Geometry check sheet. Reference: the model listing, model coordinates, mm. A direction names the side the tool comes from. Coordinates: 2 decimals unless noted, no trailing zeros. Order: outer loops, then holes, each group sorted by start corner. A loop starts at its lowest first (then second) coordinate and runs counter-clockwise, first axis right, second up. Notation, with made-up numbers: (5, -1.75) - (55, -1.75) arc R7 ccw to (55, 3.25) - close; hole circle Ø7 at (6.5, -23). An arc over 180 degrees is marked (long way). Return JSON: item names as keys, results as strings. Group by question number.
Item 1: Section check A-A on y = 12.5. Enter the section's corners in (x, z), then the cut area to 3 significant figures.
Item 2: Section check B-B on x = -63.5. Enter the section's corners in (y, z), then the cut area to 3 significant figures.
Item 3: Section check D-D on y = -45.5. Enter the section's corners in (x, z).
Item 4: Draft check along Y on faces 1 (the flat face through (-97.8, 99.7, 1.5)), 2 (the flat face through (2, 55, 0)), 3 (the flat face through (-92.82, -95.49, 1.48)). Enter one of: pulls with the +Y half, pulls with the -Y half, needs draft (parallel to the pull), parting line crosses it, or undercut.
Item 5: Section check C-C on x = 53.5. Enter the section's corners in (y, z), then the cut area to 3 significant figures.
Item 6: Scan lines: probe 1 along Y at (x, z) = (58.5, 1.8); probe 2 along X at (y, z) = (13, 1); probe 3 along Y at (x, z) = (44.4, 1.3). Record each from-to range of solid material in increasing order.
Item 7: Gauge pin test, flat ends, axial feed: pin 1 (3 mm diameter, centred on x = -44.4, y = 8, fed in from +Z); pin 2 (1.5 mm diameter, centred on y = 115, z = 2, fed in from -X); pin 3 (1.5 mm diameter, centred on y = -92, z = 1, fed in from -X); pin 4 (1 mm diameter, centred on x = -78.5, z = 1.5, fed in from +Y). Record the tip position at first contact, or that the pin passes through.
Item 8: Tool access check on faces 4 (the flat face through (2, 55, 3)), 5 (the flat face through (95.11, 97.44, 1.48)). Record the directions out of +Z, -Z, +X, -X, +Y, -Y that give a thin tool (end or side, any length) a straight path to the whole face; none if there is none.
from build123d import *

# Parameters (mm, degrees)
SKICA2_R                = 1.75
SKICA2_W                = 3
SKICA2_H                = 20
SKICA2_H_2              = 10
SKICA2_W_2              = 20
SKICA2_H_3              = 3
SKICA2_W_3              = 15
P_IDAT_VYSUNUT_M1_DEPTH = 3


with BuildPart() as part:
    # Skica2 → Přidat vysunutím1 (new body)
    with BuildSketch(Plane.XY):
        Polygon((-117.5, 80), (-77.5, 120), (77.5, 120), (117.5, 80), (117.5, -80), (77.5, -120), (-77.5, -120), (-117.5, -80), align=None)
        with Locations((58.5, 8)):
            Circle(SKICA2_R, mode=Mode.SUBTRACT)
        with Locations((44.4, 8)):
            Circle(SKICA2_R, mode=Mode.SUBTRACT)
        with Locations(Location((44.4, -8, 0), (0, 0, 180))):
            Circle(SKICA2_R, mode=Mode.SUBTRACT)
        with Locations(Location((58.5, -8, 0), (0, 0, 180))):
            Circle(SKICA2_R, mode=Mode.SUBTRACT)
        with Locations((-44.4, -8)):
            Circle(SKICA2_R, mode=Mode.SUBTRACT)
        with Locations((-58.5, -8)):
            Circle(SKICA2_R, mode=Mode.SUBTRACT)
        with Locations(Location((-58.5, 8, 0), (0, 0, 180))):
            Circle(SKICA2_R, mode=Mode.SUBTRACT)
        with Locations(Location((-44.4, 8, 0), (0, 0, 180))):
            Circle(SKICA2_R, mode=Mode.SUBTRACT)
        Polygon((-107.5, -42.5), (-107.5, 42.5), (-67.5, 42.5), (-67.5, -14), (67.5, -14), (67.5, 42.5), (107.5, 42.5), (107.5, -42.5), (107.5, -75.857864376), (73.357864376, -110), (20, -110), (10, -95), (-10, -95), (-20, -110), (-73.357864376, -110), (-107.5, -75.857864376), align=None, mode=Mode.SUBTRACT)
        with Locations((-112.5, 70)):
            Rectangle(SKICA2_W, SKICA2_H, mode=Mode.SUBTRACT)
        with Locations((-112.5, 30)):
            Rectangle(SKICA2_W, SKICA2_H, mode=Mode.SUBTRACT)
        with Locations((-112.5, 0)):
            Rectangle(SKICA2_W, SKICA2_H_2, mode=Mode.SUBTRACT)
        with Locations((-112.5, -30)):
            Rectangle(SKICA2_W, SKICA2_H, mode=Mode.SUBTRACT)
        with Locations((-112.5, -70)):
            Rectangle(SKICA2_W, SKICA2_H, mode=Mode.SUBTRACT)
        with Locations((112.5, -70)):
            Rectangle(SKICA2_W, SKICA2_H, mode=Mode.SUBTRACT)
        with Locations((112.5, -30)):
            Rectangle(SKICA2_W, SKICA2_H, mode=Mode.SUBTRACT)
        with Locations((112.5, 0)):
            Rectangle(SKICA2_W, SKICA2_H_2, mode=Mode.SUBTRACT)
        with Locations((112.5, 30)):
            Rectangle(SKICA2_W, SKICA2_H, mode=Mode.SUBTRACT)
        with Locations((112.5, 70)):
            Rectangle(SKICA2_W, SKICA2_H, mode=Mode.SUBTRACT)
        with Locations((-67.5, 115)):
            Rectangle(SKICA2_W_2, SKICA2_H_3, mode=Mode.SUBTRACT)
        with Locations((-32.5, 115)):
            Rectangle(SKICA2_W_2, SKICA2_H_3, mode=Mode.SUBTRACT)
        with Locations((0, 115)):
            Rectangle(SKICA2_W_3, SKICA2_H_3, mode=Mode.SUBTRACT)
        with Locations((32.5, 115)):
            Rectangle(SKICA2_W_2, SKICA2_H_3, mode=Mode.SUBTRACT)
        with Locations((67.5, 115)):
            Rectangle(SKICA2_W_2, SKICA2_H_3, mode=Mode.SUBTRACT)
        with Locations((67.5, -115)):
            Rectangle(SKICA2_W_2, SKICA2_H_3, mode=Mode.SUBTRACT)
        with Locations((32.5, -115)):
            Rectangle(SKICA2_W_2, SKICA2_H_3, mode=Mode.SUBTRACT)
        with Locations((0, -115)):
            Rectangle(SKICA2_W_3, SKICA2_H_3, mode=Mode.SUBTRACT)
        with Locations((-32.5, -115)):
            Rectangle(SKICA2_W_2, SKICA2_H_3, mode=Mode.SUBTRACT)
        with Locations((-67.5, -115)):
            Rectangle(SKICA2_W_2, SKICA2_H_3, mode=Mode.SUBTRACT)
        Polygon((101.168524548, -91.381727984), (88.881727984, -103.668524548), (86.76040764, -101.547204204), (99.047204204, -89.26040764), align=None, mode=Mode.SUBTRACT)
        Polygon((-86.76040764, -101.547204204), (-99.047204204, -89.26040764), (-101.168524548, -91.381727984), (-88.881727984, -103.668524548), align=None, mode=Mode.SUBTRACT)
        Polygon((86.76040764, 101.547204204), (99.047204204, 89.26040764), (101.168524548, 91.381727984), (88.881727984, 103.668524548), align=None, mode=Mode.SUBTRACT)
        Polygon((-88.881727984, 103.668524548), (-86.76040764, 101.547204204), (-99.047204204, 89.26040764), (-101.168524548, 91.381727984), align=None, mode=Mode.SUBTRACT)
    extrude(amount=P_IDAT_VYSUNUT_M1_DEPTH)


solid = part.part
Computed:
{
 "1": {"outline": "(-117.5, 0) - (-107.5, 0) - (-107.5, 3) - (-117.5, 3) - close; (-67.5, 0) - (67.5, 0) - (67.5, 3) - (-67.5, 3) - close; (107.5, 0) - (117.5, 0) - (117.5, 3) - (107.5, 3) - close", "area": "465 mm²"},
 "2": {"outline": "(-120, 0) - (-116.5, 0) - (-116.5, 3) - (-120, 3) - close; (-113.5, 0) - (-110, 0) - (-110, 3) - (-113.5, 3) - close; (-14, 0) - (113.5, 0) - (113.5, 3) - (-14, 3) - close; (116.5, 0) - (120, 0) - (120, 3) - (116.5, 3) - close", "area": "414 mm²"},
 "3": {"outline": "(-117.5, 0) - (-107.5, 0) - (-107.5, 3) - (-117.5, 3) - close; (107.5, 0) - (117.5, 0) - (117.5, 3) - (107.5, 3) - close"},
 "4": {"face 1": "pulls with the +Y half", "face 2": "needs draft", "face 3": "undercut"},
 "5": {"outline": "(-120, 0) - (-110, 0) - (-110, 3) - (-120, 3) - close; (-14, 0) - (120, 0) - (120, 3) - (-14, 3) - close", "area": "432 mm²"},
 "6": {"probe 1": "y = -120 to -116.5, -113.5 to -110, -14 to -9.75, -6.25 to 6.25, 9.75 to 113.5, 116.5 to 120", "probe 2": "x = -117.5 to -107.5, -67.5 to 67.5, 107.5 to 117.5", "probe 3": "y = -120 to -110, -14 to -9.75, -6.25 to 6.25, 9.75 to 120"},
 "7": {"pin 1": "passes through", "pin 2": "stops at x = -83.25", "pin 3": "stops at x = -106.25", "pin 4": "stops at y = 119.5"},
 "8": {"face 4": "+Z, +X, -X, +Y, -Y", "face 5": "+Z, -Z"}
}
